The listing builds one solid part. Answer for the finished solid, in the listing's coordinates (mm). A direction names the side the tool comes from. Coordinates: 2 decimals unless noted, no trailing zeros. Order: outer loops, then holes, each group sorted by start corner. A loop starts at its lowest first (then second) coordinate and runs counter-clockwise, first axis right, second up. Notation, with made-up numbers: (13, 37) -> (68, 37) arc R14 ccw to (68, 64) -> close; hole circle Ø7 at (56, 2.25). An arc over 180 degrees is marked (long way). One line per question, with ' | ' between items.
from build123d import *

# Parameters (mm, degrees)
SKICA2_W                 = 54.6
SKICA2_H                 = 4.2
SKICA2_W_2               = 25
SKICA2_H_2               = 1
P_IDAT_VYSUNUT_M2_DEPTH  = 0.4
SKICA3_R                 = 1.75
P_IDAT_VYSUNUT_M3_DEPTH  = 1.5
SKICA5_R                 = 1.9
P_IDAT_VYSUNUT_M5_DEPTH  = 2
ZKOSEN_2_SIZE            = 1.5
SKICA7_W                 = 1
SKICA7_H                 = 5
ODEBRAT_VYSUNUT_M1_DEPTH = 3.5


with BuildPart() as part:
    # Skica2 → Přidat vysunutím2 (new body)
    with BuildSketch(Plane.XY):
        Rectangle(SKICA2_W, SKICA2_H)
        Rectangle(SKICA2_W_2, SKICA2_H_2, mode=Mode.SUBTRACT)
    extrude(amount=P_IDAT_VYSUNUT_M2_DEPTH)

    # Skica3 → Přidat vysunutím3 (add)
    with BuildSketch(Plane.XY.offset(0.4)):
        with Locations((-20.3, 0)):
            Circle(SKICA3_R)
        with Locations((20.3, 0)):
            Circle(SKICA3_R)
    extrude(amount=P_IDAT_VYSUNUT_M3_DEPTH)

    # Skica5 → Přidat vysunutím5 (add)
    with BuildSketch(Plane.XY.offset(1.9)):
        with Locations((-20.3, 0)):
            Circle(SKICA5_R)
        with Locations((20.3, 0)):
            Circle(SKICA5_R)
    extrude(amount=P_IDAT_VYSUNUT_M5_DEPTH)

    # Zkosení2
    zkosen_2_edges = [part.edges().sort_by_distance(p)[0] for p in [
        (-22.2, 0, 3.9),
        (18.4, 0, 3.9),
    ]]
    chamfer(zkosen_2_edges, length=ZKOSEN_2_SIZE)

    # Skica7 → Odebrat vysunutím1 (cut)
    with BuildSketch(Plane.XY.offset(3.9)):
        with Locations((-20.3, 0)):
            Rectangle(SKICA7_W, SKICA7_H)
        with Locations((20.3, 0)):
            Rectangle(SKICA7_W, SKICA7_H)
    extrude(amount=-ODEBRAT_VYSUNUT_M1_DEPTH, mode=Mode.SUBTRACT)


solid = part.part
Item 1: Determine the mould class of faces 1 (the face through (-19, 0, 3)), 2 (the face through (-22.2, 0, 2.1)), 3 (the face through (-19.8, 0, 2)), 4 (the face through (22.2, 0, 2.1)) for opening direction X: pulls with the +X half, pulls with the -X half, needs draft (parallel to the pull), parting line crosses it, or undercut.
Computed values:
face 1: undercut | face 2: pulls with the -X half | face 3: undercut | face 4: pulls with the +X half
Item 2: For faces 5 (the face through (22.05, -0.03, 1.14)), 6 (the face through (20.8, 0, 2)), 7 (the face through (19, 0, 3)), 8 (the face through (18.55, 0.03, 1.14)), 9 (the face through (-22.05, 0.03, 1.14)), determine the directions among +Z, -Z, +X, -X, +Y, -Y from which every point of the face is accessible in a straight line to the end or side of a thin tool.
Computed values:
face 5: +X | face 6: +Z, +Y, -Y | face 7: +Z | face 8: none | face 9: -X
Item 3: Section B-B, the plane z = 1.25 is taken. Give the vertices of the cut face in (x, y).
Computed values:
outline: (-20.8, -1.68) -> (-20.8, 1.68) arc R1.75 ccw to start; (-19.8, -1.68) arc R1.75 ccw to (-19.8, 1.68) -> close; (19.8, -1.68) -> (19.8, 1.68) arc R1.75 ccw to start; (20.8, -1.68) arc R1.75 ccw to (20.8, 1.68) -> close
Item 4: Section C-C, the plane x = 15 is taken. Give the vertices of the cut face in (y, z), plus the area to 3 significant figures.
Computed values:
outline: (-2.1, 0) -> (2.1, 0) -> (2.1, 0.4) -> (-2.1, 0.4) -> close | area: 1.68 mm^2
Item 5: Each of these flat-tipped pins is pushed along its axis until it touches: pin 1 Ø1 at (y, z) = (0.5, 2.5) entering from +X; pin 2 Ø1.5 at (x, z) = (21, 2.5) entering from -Y; pin 3 Ø1 at (y, z) = (1, 2.5) entering from -X. Where does it stop, or does it pass through?
Computed values:
pin 1: stops at x = 22.2 | pin 2: stops at y = -1.83 | pin 3: stops at x = -22.13
Item 6: Section A-A, the plane x = -3.5 is taken. Give the vertices of the cut face in (y, z), plus the area to 3 significant figures.
Computed values:
outline: (-2.1, 0) -> (-0.5, 0) -> (-0.5, 0.4) -> (-2.1, 0.4) -> close; (0.5, 0) -> (2.1, 0) -> (2.1, 0.4) -> (0.5, 0.4) -> close | area: 1.28 mm^2
Item 7: Find the intervals of material crossed by L1, parallel to X at y = 0.9, z = 0.55; L2, parallel to X at y = 1.3, z = 1.25; L3, parallel to Z at x = 22.5, y = 0.5, in increasing order.
Computed values:
L1: x = -21.8 to -20.8, -19.8 to -18.8, 18.8 to 19.8, 20.8 to 21.8 | L2: x = -21.47 to -20.8, -19.8 to -19.13, 19.13 to 19.8, 20.8 to 21.47 | L3: z = 0 to 0.4
